Verification items for this drawing (mm, ordinates from the low corner). Round coordinates to 2 decimals unless told otherwise and drop trailing zeros. Loops run counter-clockwise (first coordinate to the right, second up) from the corner with the lowest first, then second, coordinate; pieces in that order, holes last. Notation, with made-up numbers: M -20.5,6 L 19.5,6 A12 ccw 19.5,24 Z; hole C -29,70.5 d6. An arc over 180 degrees is marked long. Use one line per item in the form item = value. Start each with the question number.
1. Cross-section at B-B (z = 6.25). Record the boundary of the cut face in (x, y) (1 decimal).
2. Cross-section at A-A (z = 1). Record the boundary of the cut face in (x, y) (1 decimal).
3. Go/stop test with flat-tipped pins: pin 1 (2 mm diameter, centred on y = 1.5, z = 2.5, fed in from +X); pin 2 (3 mm diameter, centred on x = 4, z = 5.5, fed in from +Y) (1 decimal). Record where each tip stops, or that it passes through.
4. Draft check along Y on the marked faces 1, 2 and 3. Enter one of: pulls with the +Y half, pulls with the -Y half, needs draft (parallel to the pull), parting line crosses it, or undercut.
5. Material ranges on line 1 (Y direction, x = 9, z = 4) (1 decimal); line 2 (Y direction, x = 6.75, z = 5) (1 decimal); line 3 (X direction, y = 8, z = 1.25), recorded low to high.
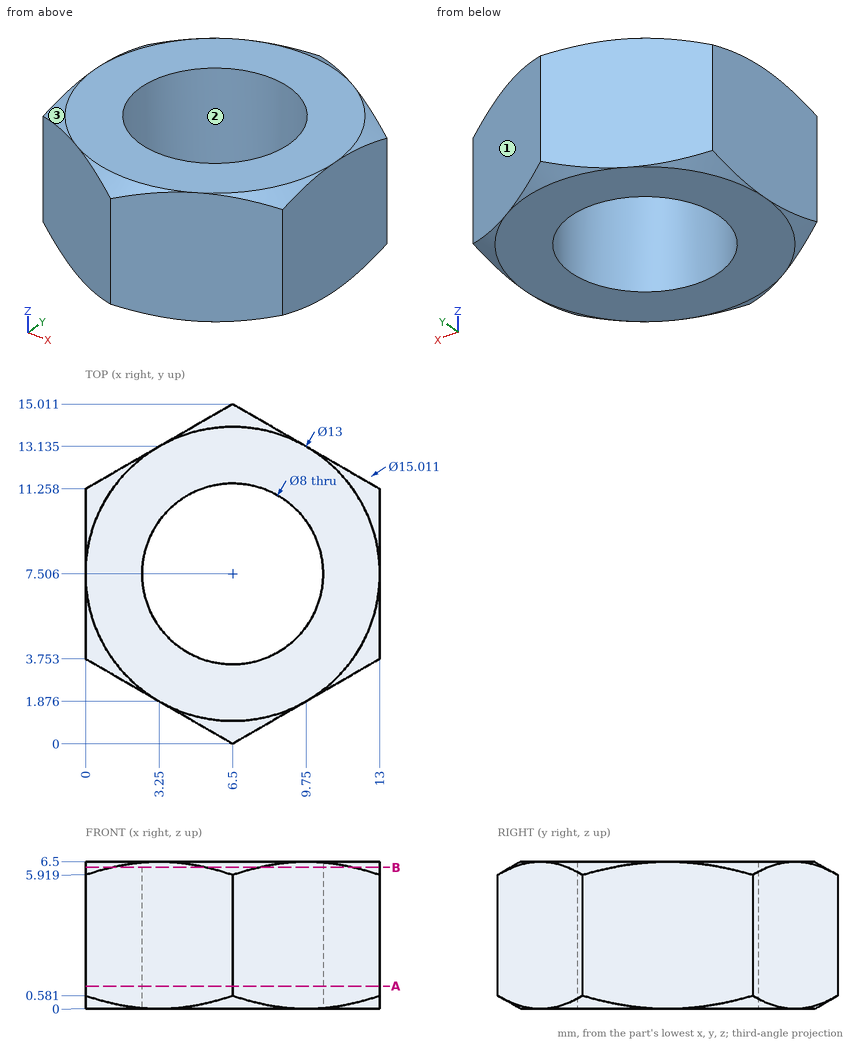
Reported:
q1.outline = M 0,5.1 A6.9 ccw 1.2,3.1 L 5.3,0.7 A6.9 ccw 7.7,0.7 L 11.8,3.1 A6.9 ccw 13,5.1 L 13,9.9 A6.9 ccw 11.8,11.9 L 7.7,14.3 A6.9 ccw 5.3,14.3 L 1.2,11.9 A6.9 ccw 0,9.9 Z; hole C 6.5,7.5 d8
q2.outline = M 0,3.8 L 6.5,0 L 13,3.8 L 13,11.3 L 6.5,15 L 0,11.3 Z; hole C 6.5,7.5 d8
q3.pin_1 = 10.83
q3.pin_2 = 14.4
q4.face_1 = pulls with the +Y half
q4.face_2 = undercut
q4.face_3 = pulls with the -Y half
q5.line_1 = 1.4 to 4.4, 10.6 to 13.6
q5.line_2 = 0.1 to 3.5, 11.5 to 14.9
q5.line_3 = 0 to 2.53, 10.47 to 13
